from build123d import *
from OCP.BRepFilletAPI import BRepFilletAPI_MakeChamfer

# Parameters (mm, degrees)
SKETCH_1_R          = 1.16
EXTRUDE_1_DEPTH     = 5
CUT_EXTRUDE_1_DEPTH = 2.1
EXTRUDE_2_DEPTH     = 2.5
EXTRUDE_3_DEPTH     = 5
CHAMFER_2_SIZE      = 0.6
CHAMFER_2_SIZE2     = 0.4738544759401763
CHAMFER_2_SIZE2_2   = 0.4738544759401755
CHAMFER_2_SIZE2_3   = 0.4397595135435583
CHAMFER_2_SIZE2_4   = 0.43975951354355786


with BuildPart() as part:
    # Sketch 1 → Extrude 1 (new, symmetric)
    with BuildSketch(Plane(origin=(0, 0, 0), x_dir=(0, 0, -1), z_dir=(1, 0, 0))):
        with BuildLine():
            Line((-18.000000000000004, 3.500000000000003), (18.000000000000004, 3.500000000000003))
            ThreePointArc((18.000000000000004, 3.500000000000003), (21.50000000000001, 3.31e-15), (18.000000000000004, -3.500000000000003))
            Line((18.000000000000004, -3.500000000000003), (-18.000000000000004, -3.500000000000003))
            ThreePointArc((-18.000000000000004, -3.500000000000003), (-21.500000000000004, 3.74e-15), (-18.000000000000004, 3.500000000000003))
        make_face()
        with Locations((18.000000000000004, 3.31e-15)):
            Circle(SKETCH_1_R, mode=Mode.SUBTRACT)
        with Locations((4, -2.2e-15)):
            Circle(SKETCH_1_R, mode=Mode.SUBTRACT)
        with Locations((-18.000000000000004, 3.31e-15)):
            Circle(SKETCH_1_R, mode=Mode.SUBTRACT)
    extrude(amount=EXTRUDE_1_DEPTH, both=True)

    # Sketch 2 → Cut-Extrude 1 (cut, symmetric)
    with BuildSketch(Plane(origin=(0, 0, 0), x_dir=(0, 0, -1), z_dir=(1, 0, 0))):
        with BuildLine():
            Line((-18.000000000000004, -3.4999999999999996), (18.000000000000004, -3.4999999999999996))
            ThreePointArc((18.000000000000004, -3.4999999999999996), (21.500000000000007, 3.31e-15), (18.000000000000004, 3.500000000000005))
            Line((18.000000000000004, 3.500000000000005), (-18.000000000000004, 3.5000000000000067))
            ThreePointArc((-18.000000000000004, 3.5000000000000067), (-21.500000000000007, 3.74e-15), (-18.000000000000004, -3.4999999999999996))
        make_face()
    extrude(amount=CUT_EXTRUDE_1_DEPTH, both=True, mode=Mode.SUBTRACT)


with BuildPart() as cut_extrude_1_piece_1:
    # of the separate pieces the step leaves, piece 1, a body of its own (cut_extrude_1_pieces)
    add(part.part.solids().sort_by_distance((-5, 3.5, 18))[0])



with BuildPart() as cut_extrude_1_piece_2:
    # of the separate pieces the step leaves, piece 2, a body of its own (cut_extrude_1_pieces)
    add(part.part.solids().sort_by_distance((2.1, 3.5, 18))[0])


with BuildPart() as cut_extrude_1_piece_1_1:
    add(cut_extrude_1_piece_1.part)

    add(cut_extrude_1_piece_2.part)  # Extrude 2 merges Cut-Extrude 1 piece 2
    # Sketch 2_4 → Extrude 2 (add, symmetric)
    with BuildSketch(Plane(origin=(0, 0, 0), x_dir=(0, 0, -1), z_dir=(1, 0, 0))):
        Polygon((-16.886363638073764, -3.3181039847171285), (-17.42832680730712, -3.500000000000003), (-1.5000000000000036, -3.4999999999999996), (-1.5000000000000053, 1.8459337107187295), align=None)
        Polygon((13.000000000000002, -3.5000000000000013), (11.000000000000002, -8.6e-16), (11.000000000000004, -3.4999999999999996), align=None)
    extrude(amount=EXTRUDE_2_DEPTH, both=True)

    # Sketch 3 → Extrude 3 (add, symmetric)
    with BuildSketch(Plane(origin=(0, 0, 0), x_dir=(0, 0, -1), z_dir=(1, 0, 0))):
        Polygon((-1.5000000000000049, -3.4999999999999996), (-13.500000000000005, -3.5000000000000027), (-11.699999999999978, -5.3000000000000025), (-3.3000000000000287, -5.300000000000003), align=None)
    extrude(amount=EXTRUDE_3_DEPTH, both=True)

    # Chamfer 2: one chamfer whose edges measure the first distance from different faces: ONE call of the kernel's chamfer builder (chamfer() names one face for all edges)
    chamfer_2_edges_1 = [cut_extrude_1_piece_1_1.edges().sort_by_distance(p)[0] for p in [
        (-5, -4.4e-16, 21.500000000000004),
        (-5, -3.500000000000003, 15.750000000000004),
        (-5, -1.2e-16, -21.50000000000001),
        (-5, 3.500000000000003, 0),
        (-5, 3.45e-15, -16.840000000000003),
        (-5, -2.06e-15, -2.84),
        (-5, 3.45e-15, 19.160000000000004),
        (5, 3.45e-15, -16.840000000000003),
        (5, -2.06e-15, -2.84),
        (5, -4.4e-16, 21.500000000000004),
        (5, -3.500000000000003, 15.750000000000004),
        (5, -1.2e-16, -21.50000000000001),
        (5, 3.500000000000003, 0),
        (5, 3.45e-15, 19.160000000000004),
        (4.4e-16, -3.4999999999999996, -11.000000000000004),
        (5, -3.500000000000003, -8.25),
        (-5, -3.500000000000003, -8.25),
        (-5, -4.400000000000002, 12.59999999999999),
        (-5, -5.3000000000000025, 7.5000000000000036),
        (-5, -4.400000000000001, 2.400000000000017),
        (5, -4.400000000000002, 12.59999999999999),
        (5, -5.3000000000000025, 7.5000000000000036),
        (5, -4.400000000000001, 2.400000000000017),
    ]]
    chamfer_2_edges_2 = [cut_extrude_1_piece_1_1.edges().sort_by_distance(p)[0] for p in [
        (4.4e-16, 1.8459337107187292, 1.5000000000000053),
    ]]
    chamfer_2_side_2 = [cut_extrude_1_piece_1_1.faces().sort_by_distance(p)[0] for p in [
        (1e-17, -0.827033144640636, 1.500000000000005),
    ]]
    chamfer_2_edges_3 = [cut_extrude_1_piece_1_1.edges().sort_by_distance(p)[0] for p in [
        (4.4e-16, -3.5000000000000013, 17.42832680730712),
    ]]
    chamfer_2_side_3 = [cut_extrude_1_piece_1_1.faces().sort_by_distance(p)[0] for p in [
        (-2e-17, -0.8270331446406359, 9.464163403653561),
    ]]
    chamfer_2_edges_4 = [cut_extrude_1_piece_1_1.edges().sort_by_distance(p)[0] for p in [
        (4.4e-16, -3.5000000000000013, -13.000000000000002),
    ]]
    chamfer_2_side_4 = [cut_extrude_1_piece_1_1.faces().sort_by_distance(p)[0] for p in [
        (4.780853929991888, -3.500000000000003, -8.25),
    ]]
    chamfer_2_edges_5 = [cut_extrude_1_piece_1_1.edges().sort_by_distance(p)[0] for p in [
        (-4.4e-16, -8.6e-16, -11.000000000000002),
    ]]
    chamfer_2_side_5 = [cut_extrude_1_piece_1_1.faces().sort_by_distance(p)[0] for p in [
        (-1e-17, -1.7500000000000009, -12.000000000000002),
    ]]
    chamfer_2 = BRepFilletAPI_MakeChamfer(cut_extrude_1_piece_1_1.part.solid().wrapped)
    for e in chamfer_2_edges_1:
        chamfer_2.Add(CHAMFER_2_SIZE, e.wrapped)
    for e in chamfer_2_edges_2:
        chamfer_2.Add(CHAMFER_2_SIZE, CHAMFER_2_SIZE2, e.wrapped, chamfer_2_side_2[0].wrapped)  # the first distance lies on this face
    for e in chamfer_2_edges_3:
        chamfer_2.Add(CHAMFER_2_SIZE, CHAMFER_2_SIZE2_2, e.wrapped, chamfer_2_side_3[0].wrapped)  # the first distance lies on this face
    for e in chamfer_2_edges_4:
        chamfer_2.Add(CHAMFER_2_SIZE, CHAMFER_2_SIZE2_3, e.wrapped, chamfer_2_side_4[0].wrapped)  # the first distance lies on this face
    for e in chamfer_2_edges_5:
        chamfer_2.Add(CHAMFER_2_SIZE, CHAMFER_2_SIZE2_4, e.wrapped, chamfer_2_side_5[0].wrapped)  # the first distance lies on this face
    add(Compound.cast(chamfer_2.Shape()), mode=Mode.REPLACE)


solid = cut_extrude_1_piece_1_1.part
The model under review builds one solid part; all positions refer to its coordinate system, in mm. A direction names the side the tool comes from. Round coordinates to 2 decimals unless told otherwise and drop trailing zeros. Write each loop counter-clockwise with the first axis right and the second up, starting at its lowest first coordinate (ties: lowest second). Pieces come first, ordered by that corner, then holes. Notation, with made-up numbers: M 4.5,8.25 L 32.5,8.25 A20 ccw 32.5,17.25 Z; hole C -7,-27 d4. An arc over 180 degrees is marked long. Use a Markdown table: item, result. Add a question column.
Q1. Insertion check: pin 1 (2 mm diameter, centred on y = 0, z = -4, fed in from -X); pin 2 (1 mm diameter, centred on x = -0.5, z = 15.5, fed in from +Y) (3 decimals); pin 3 (1.3 mm diameter, centred on x = -1.5, z = 16.5, fed in from -Y); pin 4 (5 mm diameter, centred on x = -2.5, y = -3, fed in from +Z). Each pin has a flat end and moves straight along its axis. Give the tip position at first contact, or say it passes through.
Q2. To check wall thickness, follow line 1 (X direction, y = 0, z = -7); line 2 (Z direction, x = 4.5, y = -0.5); line 3 (Z direction, x = 4.5, y = 1). State the ranges of each line that lie inside material, in increasing order.
Q3. We need section C-C, the plane x = -3.5. State the section outline as (y, z) points.
Q4. We need section B-B, the plane z = -10. State the section outline as (x, y) points.
Q5. Machinability: for faces 1 (the face through (0.03, -1.84, -12.05)), 2 (the face through (0, -5.3, 8)), 3 (the face through (0, -2, -11)), which of the approach directions +Z, -Z, +X, -X, +Y, -Y give a long, thin tool a straight path to every point of the face, cutting with its end or side? Answer none if there is none.
Q6. We need section D-D, the plane z = -4. State the section outline as (x, y) points, plus the area to 3 significant figures.
Q7. The part is to be moulded in two halves that separate along X. For faces 4 (the face through (-4.8, 0.1, -21.1)), 5 (the face through (3.234, 0.348, 16.894)), 6 (the face through (2.1, 0, 0)), 7 (the face through (5, 0, 0)), say which applies: pulls with the +X half, pulls with the -X half, needs draft (parallel to the pull), parting line crosses it, or undercut.
Q8. We need section A-A, the plane x = 1.5. State the section outline as (y, z) points.
Findings below:
| question | item | result |
|---|---|---|
| 1 | pin 1 | passes through |
| 1 | pin 2 | stops at y = -2.685 |
| 1 | pin 3 | stops at y = -3.5 |
| 1 | pin 4 | stops at z = 21.46 |
| 2 | line 1 | x = -5 to -2.1, 2.1 to 5 |
| 2 | line 2 | z = -21.36 to -19.16, -16.84 to -5.16, -2.84 to 16.84, 19.16 to 21.36 |
| 2 | line 3 | z = -21.25 to -18.77, -17.23 to -4.77, -3.23 to 17.23, 18.77 to 21.25 |
| 3 | outline | M -5.3,3.3 L -3.5,1.5 L -3.5,-18 A3.5 ccw 3.5,-18 L 3.5,18 A3.5 ccw -3.5,18 L -3.5,13.5 L -5.3,11.7 Z; hole C 0,-18 d2.32; hole C 0,-4 d2.32; hole C 0,18 d2.32 |
| 4 | outline | M -5,-2.9 L -4.4,-3.5 L -2.1,-3.5 L -2.1,3.5 L -4.4,3.5 L -5,2.9 Z; M 2.1,-3.5 L 4.4,-3.5 L 5,-2.9 L 5,2.9 L 4.4,3.5 L 2.1,3.5 Z |
| 5 | face 1 | -Z, +Y |
| 5 | face 2 | +Z, -Z, +X, -X, -Y |
| 5 | face 3 | +Y, -Y |
| 6 | outline | M -5,-2.9 L -4.4,-3.5 L -2.1,-3.5 L -2.1,-1.16 L -4.4,-1.16 L -5,-1.76 Z; M -5,1.76 L -4.4,1.16 L -2.1,1.16 L -2.1,3.5 L -4.4,3.5 L -5,2.9 Z; M 2.1,-3.5 L 4.4,-3.5 L 5,-2.9 L 5,-1.76 L 4.4,-1.16 L 2.1,-1.16 Z; M 2.1,1.16 L 4.4,1.16 L 5,1.76 L 5,2.9 L 4.4,3.5 L 2.1,3.5 Z |
| 6 | area | 25.7 mm² |
| 7 | face 4 | pulls with the -X half |
| 7 | face 5 | needs draft |
| 7 | face 6 | undercut |
| 7 | face 7 | pulls with the +X half |
| 8 | outline | M -5.3,3.3 L -3.5,1.5 L 1.25,1.5 L 1.7,1.95 L -3.31,16.86 L -3.5,16.95 L -3.5,13.5 L -5.3,11.7 Z; M -3.5,-12.4 L -3.12,-12.78 L -0.52,-11.3 L -0.44,-11 L -2.9,-11 L -3.5,-11.6 Z |
